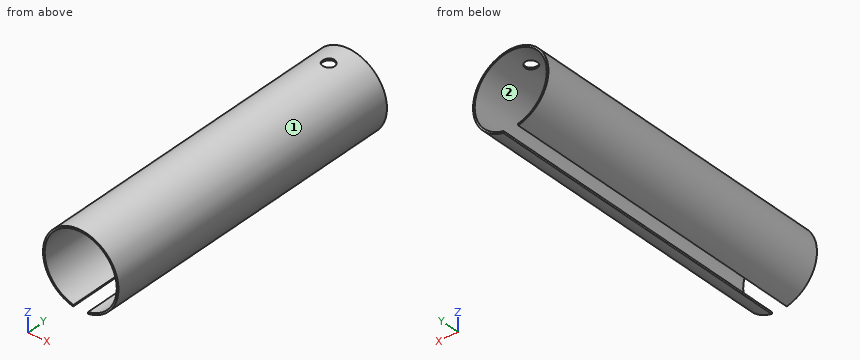
```python
from build123d import *

# Parameters (mm, degrees)
EXTRUDE_1_DEPTH     = 13
SKETCH_2_R          = 0.25
CUT_EXTRUDE_1_DEPTH = 2.57


with BuildPart() as part:
    # Эскиз1 → Бобышка-Вытянуть1 (new body)
    with BuildSketch(Plane(origin=(0, 0, 0), x_dir=(1, 0, 0), z_dir=(0, 1, 0))):
        with BuildLine():
            Line((-0.314, 1.538279558), (-0.3, 1.469693846))
            ThreePointArc((-0.3, 1.469693846), (0, -1.5), (0.3, 1.469693846))
            Line((0.3, 1.469693846), (0.314, 1.538279558))
            ThreePointArc((0.314, 1.538279558), (0, -1.57), (-0.314, 1.538279558))
        make_face()
    extrude(amount=EXTRUDE_1_DEPTH)

    # Эскиз2 → Вырез-Вытянуть1 (cut, through all)
    with BuildSketch(Plane.XY):
        with Locations((0, 12)):
            Circle(SKETCH_2_R)
    extrude(amount=CUT_EXTRUDE_1_DEPTH, mode=Mode.SUBTRACT)


solid = part.part
```
Input: part model. Units: mm. Frame: model coordinates. Face numbers are marked on the shaded views. Coordinates: 2 decimals unless noted, no trailing zeros. Order: outer loops, then holes, each group sorted by start corner. A loop starts at its lowest first (then second) coordinate and runs counter-clockwise, first axis right, second up. Notation, with made-up numbers: (-39, 21.5) - (17, 21.5) arc R25 ccw to (17, 48.5) - close; hole circle Ø1 at (-36.75, 79.5). An arc over 180 degrees is marked (long way). Return JSON: item names as keys, results as strings.
Q1. Draft query along X for the marked faces 1 and 2. Return one class per face: +X half, -X half, draft (parallel to the pull), parting line (faces both ways), or undercut.
The answers:
{"face 1": "parting line", "face 2": "undercut"}
Q2. First-contact query: pin 1 (1.5 mm diameter, centred on x = -1, y = 10, fed in from -Z); pin 2 (1.8 mm diameter, centred on x = 0, z = 0, fed in from +Y). Flat tips, straight axial feed; report the tip coordinate or a pass-through.
The answers:
{"pin 1": "stops at z = -1.54", "pin 2": "passes through"}
Q3. Cut plane B-B (z = 0). Return loops of the section in (x, y), then the cut area to 3 significant figures.
The answers:
{"outline": "(-1.57, 0) - (-1.5, 0) - (-1.5, 13) - (-1.57, 13) - close; (1.5, 0) - (1.57, 0) - (1.57, 13) - (1.5, 13) - close", "area": "1.82 mm2"}
Q4. Cut plane A-A (x = 0). Return loops of the section in (y, z).
The answers:
{"outline": "(0, 1.5) - (11.75, 1.5) - (11.75, 1.57) - (0, 1.57) - close; (12.25, 1.5) - (13, 1.5) - (13, 1.57) - (12.25, 1.57) - close"}
Q5. Cut plane C-C (y = 2.5). Return loops of the section in (x, z), then the cut area to 3 significant figures.
The answers:
{"outline": "(-0.31, -1.54) - (-0.3, -1.47) arc R1.5 cw (long way) to (0.3, -1.47) - (0.31, -1.54) arc R1.57 ccw (long way) to start", "area": "0.632 mm2"}
